Design review of the part built by this model. Coordinates are the model's own, in mm. Face numbers are marked on the shaded views. A direction names the side the tool comes from. Round coordinates to 2 decimals unless told otherwise and drop trailing zeros. Loops run counter-clockwise (first coordinate to the right, second up) from the corner with the lowest first, then second, coordinate; pieces in that order, holes last. Notation, with made-up numbers: (-12, -28) - (42, -28) arc R31 ccw to (42, -4) - close; hole circle Ø7 at (63.5, -5.5). An arc over 180 degrees is marked (long way). Answer as CSV lines item,"result". Start each with the question number.
(1) Consider section B-B (z = 32.5). Give the boundary of the cut face in (x, y).
(2) For the marked faces 5, 6 and 7, list the 3-axis set-ups (+Z, -Z, +X, -X, +Y, -Y) from which the entire face can be reached by the end or side of a thin tool; tool diameter is ignored.
(3) Wall thickness on L1, parallel to Z at x = -15, y = 26; L2, parallel to Y at x = -22, z = 26; L3, parallel to X at y = 30, z = 23.5: over which ranges is each line inside the solid? List them lowest first.
(4) Mouldability with a two-part tool opening along X and no side actions: class the marked faces 1, 2, 3 and 4 as released by +X, released by -X, zero draft, split by the parting line, or undercut.
(5) For P1, Ø3, axis at x = -21, y = -15, coming from the +Z side; P2, Ø12, axis at x = 42, z = 37.5, coming from the -Y side; P3, Ø1, axis at y = -17, z = 22.5, coming from the +X side; P4, Ø10, axis at x = 17, y = 26, coming from the -Z side, all flat-tipped, find the tip position at first contact; note any pin that passes through.
(6) Consider section C-C (x = -19). Give the boundary of the cut face in (y, z), and give its area (3 significant figures).
(7) Consider section D-D (z = 14). Give the boundary of the cut face in (x, y).
(8) Consider section A-A (y = 7.5). Give the boundary of the cut face in (x, z).
from build123d import *

# Parameters (mm, degrees)
F1_DEPTH = 25
F3_DEPTH = 25
F4_R     = 11.23983
F5_DEPTH = 25


with BuildPart() as f1:
    # F0 (on Top) → F1 (new body)
    with BuildSketch(Plane.XY):
        Polygon((23.434135, 40.589113), (-23.434135, 40.589113), (-46.86827, 0), (-23.434135, -40.589113), (23.434135, -40.589113), (46.86827, 0), align=None)
    extrude(amount=F1_DEPTH)

    # F2 (on face) → F3 (join)
    with BuildSketch(Plane.XY.offset(25)):
        with BuildLine():
            Line((46.86827, 0), (23.434135, 40.589113))
            ThreePointArc((23.434135, 40.589113), (14.856646, 8.577489), (46.86827, 0))
        make_face()
        with BuildLine():
            ThreePointArc((46.86827, 0), (55.445759, 8.577489), (58.585338, 20.294556))
            ThreePointArc((58.585338, 20.294556), (46.86827, 40.589113), (23.434135, 40.589113))
            Line((23.434135, 40.589113), (46.86827, 0))
        make_face()
    extrude(amount=F3_DEPTH)

    # F4 (on face) → F5 (join)
    with BuildSketch(Plane.XY.offset(25)):
        with Locations((-21.189533, 0)):
            Circle(F4_R)
    extrude(amount=F5_DEPTH)


solid = f1.part
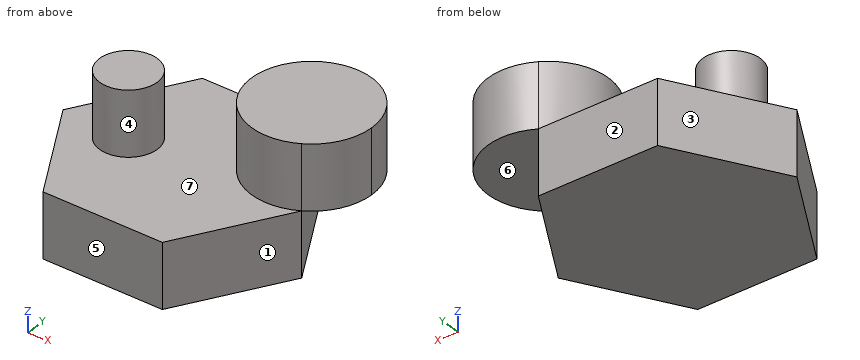
Determined:
1,outline,"circle Ø22.48 at (-21.19, 0); (46.87, 0) arc R23.43 ccw to (58.59, 20.29) arc R23.43 ccw (long way) to start"
2,face 5,"+Z, -Z, +X, -X, -Y"
2,face 6,"-Z, +X, +Y"
2,face 7,"+Z"
3,L1,"z = 0 to 25"
3,L2,"y = -11.21 to 11.21"
3,L3,"x = -29.55 to 29.55"
4,face 1,"released by +X"
4,face 2,"zero draft"
4,face 3,"released by -X"
4,face 4,"undercut"
5,P1,"stops at z = 25"
5,P2,"stops at y = -3.12"
5,P3,"stops at x = 37.34"
5,P4,"stops at z = 0"
6,outline,"(-40.59, 0) - (40.59, 0) - (40.59, 25) - (11.02, 25) - (11.02, 50) - (-11.02, 50) - (-11.02, 25) - (-40.59, 25) - close"
6,area,"2,580 mm^2"
7,outline,"(-46.87, 0) - (-23.43, -40.59) - (23.43, -40.59) - (46.87, 0) - (23.43, 40.59) - (-23.43, 40.59) - close"
8,outline,"(-42.54, 0) - (42.54, 0) - (42.54, 25) - (54.78, 25) - (54.78, 50) - (15.52, 50) - (15.52, 25) - (-12.82, 25) - (-12.82, 50) - (-29.56, 50) - (-29.56, 25) - (-42.54, 25) - close"
